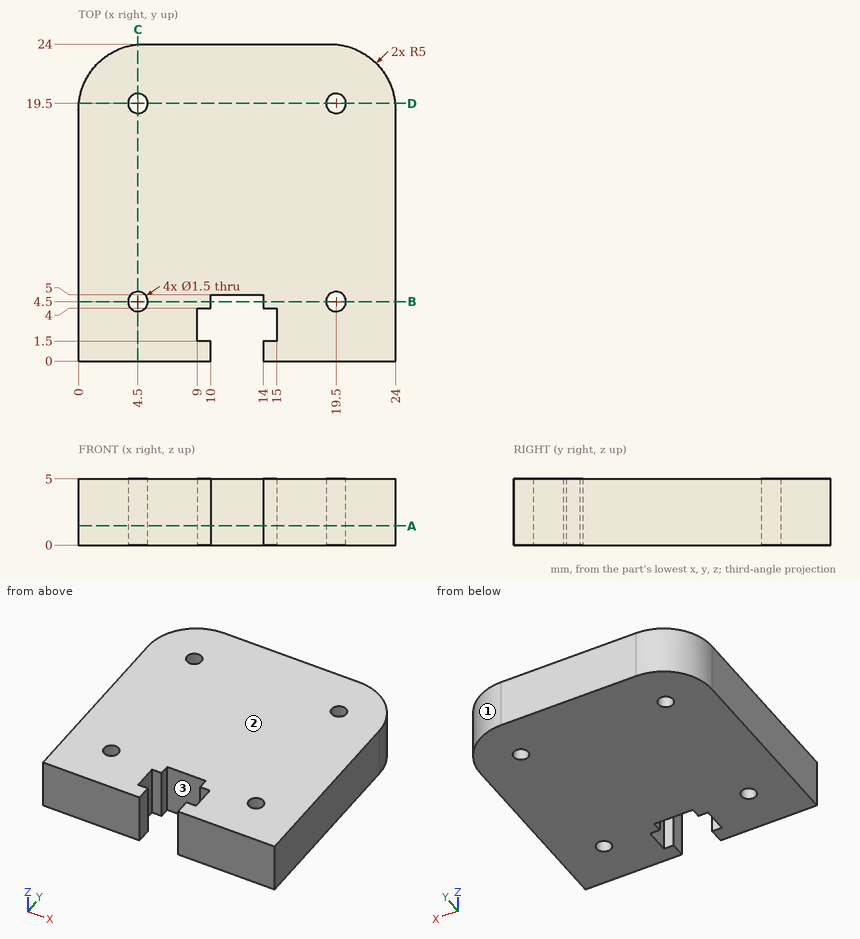
Geometry: see drawing. Coordinates: mm, zero at the bounding-box minimum. Coordinates: 2 decimals unless noted, no trailing zeros. Loops run counter-clockwise (first coordinate to the right, second up) from the corner with the lowest first, then second, coordinate; pieces in that order, holes last.
(1) Pull-direction query (X, two-part tool) for the marked faces 1, 2 and 3; classes: released by +X, released by -X, zero draft, split by the parting line, or undercut.
(2) First-contact query: pin 1 Ø3 at (x, z) = (2.5, 3) entering from +Y. Flat tip, straight axial feed; report the tip coordinate or a pass-through.
(3) Section C-C on x = 4.5. Return the cut outline in (y, z).
(4) Section D-D on y = 19.5. Return the cut outline in (x, z).
(5) Section A-A on z = 1.45. Return the cut outline in (x, y), then the cut area to 3 significant figures.
(6) Material intervals for probe 1 along Y at (x, z) = (19.5, 2.6); probe 2 along Y at (x, z) = (12, 2.6); probe 3 along X at (y, z) = (21.75, 0.3), sorted ascending.
(7) Section B-B on y = 4.5. Return the cut outline in (x, z), then the cut area to 3 significant figures.
Data:
1. face 1: released by +X
1. face 2: zero draft
1. face 3: undercut
2. pin 1: stops at y = 23.9
3. outline: (0, 0) - (3.75, 0) - (3.75, 5) - (0, 5) - close; (5.25, 0) - (18.75, 0) - (18.75, 5) - (5.25, 5) - close; (20.25, 0) - (23.97, 0) - (23.97, 5) - (20.25, 5) - close
4. outline: (0.03, 0) - (3.75, 0) - (3.75, 5) - (0.03, 5) - close; (5.25, 0) - (18.75, 0) - (18.75, 5) - (5.25, 5) - close; (20.25, 0) - (23.97, 0) - (23.97, 5) - (20.25, 5) - close
5. outline: (0, 0) - (10, 0) - (10, 1.5) - (9, 1.5) - (9, 4) - (10, 4) - (10, 5) - (14, 5) - (14, 4) - (15, 4) - (15, 1.5) - (14, 1.5) - (14, 0) - (24, 0) - (24, 19) arc R5 ccw to (19, 24) - (5, 24) arc R5 ccw to (0, 19) - close; hole circle Ø1.5 at (4.5, 4.5); hole circle Ø1.5 at (4.5, 19.5); hole circle Ø1.5 at (19.5, 4.5); hole circle Ø1.5 at (19.5, 19.5)
5. area: 533 mm2
6. probe 1: y = 0 to 3.75, 5.25 to 18.75, 20.25 to 23.97
6. probe 2: y = 5 to 24
6. probe 3: x = 0.82 to 23.18
7. outline: (0, 0) - (3.75, 0) - (3.75, 5) - (0, 5) - close; (5.25, 0) - (10, 0) - (10, 5) - (5.25, 5) - close; (14, 0) - (18.75, 0) - (18.75, 5) - (14, 5) - close; (20.25, 0) - (24, 0) - (24, 5) - (20.25, 5) - close
7. area: 85.0 mm2
